Input: part model. Units: mm. Frame: model coordinates. Face numbers are marked on the shaded views. A direction names the side the tool comes from. Give positions to 0.01 mm unless a question says otherwise; leave off trailing zeros. Loops run counter-clockwise (first coordinate to the right, second up) from the corner with the lowest first, then second, coordinate; pieces in that order, holes last. Notation, with made-up numbers: (45, -29.75) - (102, -29.75) arc R23 ccw to (102, -4.75) - close; hole circle Ø6 at (73, 54.5). An arc over 180 degrees is marked (long way). Answer as a JSON object with one key per item and string values.
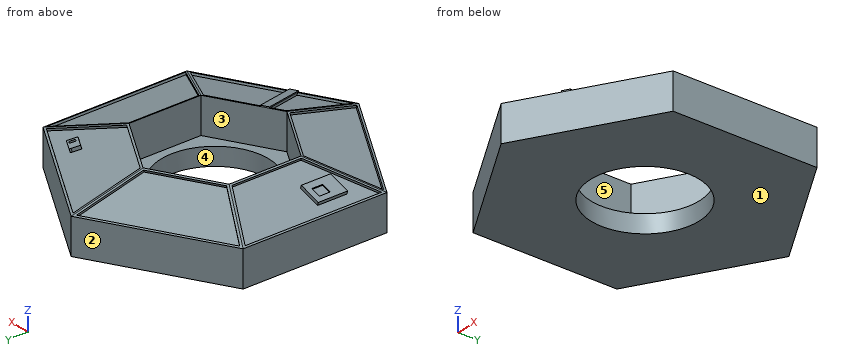
from build123d import *

# Parameters (mm, degrees)
F0_R      = 9.525
F1_DEPTH  = 6.35
F2_R      = 9.525
F3_DEPTH  = 3.175
F8_DEPTH  = 6.35
F9_W      = 3.8866475224
F9_H      = 5.1821961533
F9_W_2    = 1.7273994163
F9_H_2    = 1.9001385663
F10_DEPTH = 0.1905
F12_DEPTH = 0.1905
F13_DEPTH = 0.381
F15_DEPTH = 0.381
F17_DEPTH = 0.381
F18_W     = 3.8866475224
F18_H     = 5.1821961533
F19_DEPTH = 0.381
F21_DEPTH = 0.381
F23_DEPTH = 0.381
F25_DEPTH = 0.635


# Not quite as in the source:
# - a feature names something its author has since deleted; it is built from what else it names


with BuildPart() as f1:
    # F0 (on Top) → F1 (new body)
    with BuildSketch(Plane.XY):
        Polygon((21.9970452561, 12.7), (0, 25.4), (-21.9970452561, 12.7), (-21.9970452561, -12.7), (0, -25.4), (21.9970452561, -12.7), align=None)
        Polygon((-10.9985226281, 6.35), (0, 12.7), (10.9985226281, 6.35), (10.9985226281, -6.35), (0, -12.7), (-10.9985226281, -6.35), align=None, mode=Mode.SUBTRACT)
        Polygon((10.9985226281, 6.35), (0, 12.7), (-10.9985226281, 6.35), (-10.9985226281, -6.35), (0, -12.7), (10.9985226281, -6.35), align=None)
        Circle(F0_R, mode=Mode.SUBTRACT)
    extrude(amount=F1_DEPTH)

    # F2 (on face) → F3 (join)
    with BuildSketch(Plane.XY.offset(6.35)):
        Polygon((-10.9985226281, 6.35), (-10.9985226281, -6.35), (0, -12.7), (10.9985226281, -6.35), (10.9985226281, 6.35), (0, 12.7), align=None)
        Circle(F2_R, mode=Mode.SUBTRACT)
    extrude(amount=F3_DEPTH)

    # F4 (on face) → F6 section 0
    with BuildSketch(Plane.XY.offset(6.35)):
        Polygon((0, -25.4), (21.9970452561, -12.7), (21.9970452561, 12.7), (0, 25.4), (-21.9970452561, 12.7), (-21.9970452561, -12.7), align=None)
    # F5 (on face) → F6 section 1
    with BuildSketch(Plane.XY.offset(9.525)):
        Polygon((0, -12.7), (10.9985226281, -6.35), (10.9985226281, 6.35), (0, 12.7), (-10.9985226281, 6.35), (-10.9985226281, -6.35), align=None)
    loft()

    # F8 (cut): a face of the model
    f8_faces = [f1.faces().sort_by_distance(p)[0] for p in [
        (0, 0, 9.525),
    ]]
    extrude(f8_faces, amount=-F8_DEPTH, mode=Mode.SUBTRACT)

    # F9 (on face) → F10 (join)
    with BuildSketch(Plane(origin=(-3.3841608086, 0, 11.7230769231), x_dir=(0.9607689228, 0, 0.2773500981), z_dir=(-0.2773500981, 0, 0.9607689228))):
        with Locations((-14.8150864989, -5.1390115405)):
            Rectangle(F9_W, F9_H)
        with Locations((-14.9446423166, -4.4480519136)):
            Rectangle(F9_W_2, F9_H_2, mode=Mode.SUBTRACT)
    extrude(amount=F10_DEPTH)

    # F11 (on face) → F12 (join)
    with BuildSketch(Plane(origin=(1.6920804043, -2.9307692308, 11.7230769231), x_dir=(0.9903379377, 0.0336336397, -0.1345345588), z_dir=(0.1386750491, -0.2401922307, 0.9607689228))):
        Polygon((1.7312151801, -8.1025979269), (0.5512164028, -8.7571434803), (6.1041303172, -18.7678014037), (7.2841290946, -18.1132558503), align=None)
    extrude(amount=F12_DEPTH)

    # F7 (on face) → F13 (cut)
    with BuildSketch(Plane(origin=(3.3841608086, 0, 11.7230769231), x_dir=(0.9607689228, 0, -0.2773500981), z_dir=(0.2773500981, 0, 0.9607689228))):
        Polygon((8.1792790536, 6.2004337374), (8.1792790536, -6.2004337374), (19.1189043532, -12.2686460377), (19.1189043532, 12.2686460377), align=None)
    extrude(amount=-F13_DEPTH, mode=Mode.SUBTRACT)

    # F14 (on face) → F15 (cut)
    with BuildSketch(Plane(origin=(1.6920804043, 2.9307692308, 11.7230769231), x_dir=(0.9903379377, -0.0336336397, -0.1345345588), z_dir=(0.1386750491, 0.2401922307, 0.9607689228))):
        Polygon((-1.3275888968, 22.4544873413), (-1.3275888968, 10.2350073173), (9.3858632247, 4.2922533233), (19.7524424685, 10.7613898066), align=None)
    extrude(amount=-F15_DEPTH, mode=Mode.SUBTRACT)

    # F16 (on face) → F17 (cut)
    with BuildSketch(Plane(origin=(-1.6920804043, 2.9307692308, 11.7230769231), x_dir=(0.9903379377, 0.0336336397, 0.1345345588), z_dir=(-0.1386750491, 0.2401922307, 0.9607689228))):
        Polygon((-19.7524424685, 10.7613898066), (-9.3858632247, 4.2922533233), (1.3275888968, 10.2350073173), (1.3275888968, 22.4544873413), align=None)
    extrude(amount=-F17_DEPTH, mode=Mode.SUBTRACT)

    # F18 (on face) → F19 (cut)
    with BuildSketch(Plane(origin=(-3.3841608086, 0, 11.7230769231), x_dir=(0.9607689228, 0, 0.2773500981), z_dir=(-0.2773500981, 0, 0.9607689228))):
        Polygon((-8.3062790536, 6.1256506061), (-18.9919043532, 12.0529690566), (-18.9919043532, -12.0529690566), (-8.3062790536, -6.1256506061), align=None)
        with Locations((-14.8150864989, -5.1390115405)):
            Rectangle(F18_W, F18_H, mode=Mode.SUBTRACT)
    extrude(amount=-F19_DEPTH, mode=Mode.SUBTRACT)

    # F20 (on face) → F21 (cut)
    with BuildSketch(Plane(origin=(-1.6920804043, -2.9307692308, 11.7230769231), x_dir=(0.9903379377, -0.0336336397, 0.1345345588), z_dir=(-0.1386750491, -0.2401922307, 0.9607689228))):
        Polygon((1.3275888968, -22.4544873413), (1.3275888968, -10.2350073173), (-9.3858632247, -4.2922533233), (-19.7524424685, -10.7613898066), align=None)
    extrude(amount=-F21_DEPTH, mode=Mode.SUBTRACT)

    # F22 (on face) → F23 (cut)
    with BuildSketch(Plane(origin=(1.6920804043, -2.9307692308, 11.7230769231), x_dir=(0.9903379377, 0.0336336397, -0.1345345588), z_dir=(0.1386750491, -0.2401922307, 0.9607689228))):
        Polygon((9.3858632247, -4.2922533233), (1.9160273264, -8.4357727618), (7.0993169483, -17.7800810155), (19.7524424685, -10.7613898066), align=None)
        Polygon((5.9193181709, -18.4346265688), (0.736028549, -9.0903183152), (-1.3275888968, -10.2350073173), (-1.3275888968, -22.4544873413), align=None)
    extrude(amount=-F23_DEPTH, mode=Mode.SUBTRACT)

    # F24 (on face) → F25 (join)
    with BuildSketch(Plane(origin=(1.6392452106, 2.8392559909, 11.3570239635), x_dir=(0.9903379377, -0.0336336397, -0.1345345588), z_dir=(0.1386750491, 0.2401922307, 0.9607689228))):
        Polygon((14.1548511611, 11.4204940112), (12.0419776672, 12.5925053529), (11.9030368338, 12.3420262032), (11.2298887321, 11.1284912051), (13.3427622261, 9.9564798634), align=None)
        Polygon((12.6895471254, 10.7929574783), (13.1615737293, 11.6439155403), (13.6242877942, 11.3872479577), (13.1522611902, 10.5362898958), align=None, mode=Mode.SUBTRACT)
    extrude(amount=F25_DEPTH)


solid = f1.part
Item 1: Cut plane B-B (z = 1.25). Return loops of the section in (x, y) (3 decimals).
Geometry check:
{"outline": "(-21.997, -12.7) - (0, -25.4) - (21.997, -12.7) - (21.997, 12.7) - (0, 25.4) - (-21.997, 12.7) - close; hole circle Ø19.05 at (0, 0)"}
Item 2: Access query for the marked faces 4 and 5. Directions: +Z, -Z, +X, -X, +Y, -Y. A direction counts if a zero-diameter tool reaches every point of the face in a straight line with its end or side. Return the directions, or none.
Geometry check:
{"face 4": "+Z, -Z", "face 5": "+Z"}
Item 3: Mould query, pull axis Y, two halves, no side actions, for the marked faces 1, 2 and 3. Classes: released by +Y, released by -Y, zero draft, split by the parting line, or undercut.
Geometry check:
{"face 1": "zero draft", "face 2": "released by +Y", "face 3": "undercut"}
Item 4: Cut plane A-A (z = 4.5). Return loops of the section in (x, y), then the cut area to 3 significant figures.
Geometry check:
{"outline": "(-22, -12.7) - (0, -25.4) - (22, -12.7) - (22, 12.7) - (0, 25.4) - (-22, 12.7) - close; hole (-11, -6.35) - (0, -12.7) - (11, -6.35) - (11, 6.35) - (0, 12.7) - (-11, 6.35) - close", "area": "1,260 mm2"}
Item 5: Contact query for flat-ended pins moving along their axis: P1, Ø6, axis at x = -16, y = 17, coming from the +Z side; P2, Ø1.8, axis at x = -18.5, z = 8, coming from the -Y side; P3, Ø0.5, axis at x = -18, z = 7.5, coming from the -Y side. Output: stop coordinate, or through.
Geometry check:
{"P1": "stops at z = 6.61", "P2": "stops at y = -11.3", "P3": "stops at y = -10.94"}
Item 6: Material intervals for line 1 (X direction, y = 0, z = 2.3) (3 decimals); line 2 (X direction, y = 1, z = 5); line 3 (Y direction, x = 0, z = 1.9) (3 decimals), sorted ascending. Write a range as [from, to].
Geometry check:
{"line 1": "x = [-21.997, -9.525], [9.525, 21.997]", "line 2": "x = [-22, -11], [11, 22]", "line 3": "y = [-25.4, -9.525], [9.525, 25.4]"}
